Verification items for the finished model (mm, model axes). Face numbers are marked on the shaded views. A direction names the side the tool comes from. Coordinates: 2 decimals unless noted, no trailing zeros. Order: outer loops, then holes, each group sorted by start corner. A loop starts at its lowest first (then second) coordinate and runs counter-clockwise, first axis right, second up. Notation, with made-up numbers: (78, 26) -> (115, 26) arc R6 ccw to (115, 31) -> close; hole circle Ø6 at (56.25, -22.75). An arc over 180 degrees is marked (long way). Write item = value, one per line. Start each with the question number.
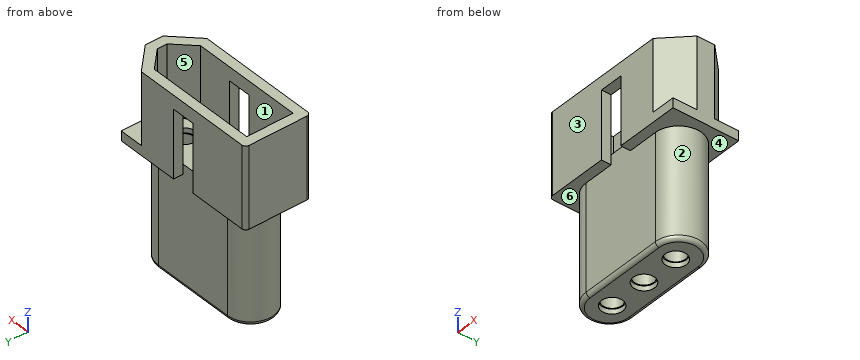
from build123d import *

# Parameters (mm, degrees)
BOSS_EXTRUDE1_DEPTH = 10.668
SKETCH2_R           = 1.27
BOSS_EXTRUDE2_DEPTH = 15.6591
BOSS_EXTRUDE3_START = -1.27
BOSS_EXTRUDE3_DEPTH = 1.27
SKETCH4_R           = 1.397
CUT_EXTRUDE1_DEPTH  = 0.635
CUT_EXTRUDE2_START  = -0.635
SKETCH5_R           = 1.397
CUT_EXTRUDE2_DEPTH  = 0.635
SKETCH6_W           = 3.048
SKETCH6_H           = 1.27
CUT_EXTRUDE3_DEPTH  = 8.89
FILLET1_R           = 0.508


# Read off the part's stored shape, not the designer's step: Boss-Extrude3
with BuildPart() as part:
    # Sketch1 → Boss-Extrude1 (new body)
    with BuildSketch(Plane.XY):
        with BuildLine():
            Line((6.622051224, 4.318), (-9.271, 4.318))
            ThreePointArc((-9.271, 4.318), (-9.630210245, 4.169210245), (-9.779, 3.81))
            Line((-9.779, 3.81), (-9.779, -3.81))
            ThreePointArc((-9.779, -3.81), (-9.630210245, -4.169210245), (-9.271, -4.318))
            Line((-9.271, -4.318), (6.622051224, -4.318))
            Line((6.622051224, -4.318), (9.779, -1.161051224))
            Line((9.779, -1.161051224), (9.779, 1.161051224))
            Line((9.779, 1.161051224), (6.622051224, 4.318))
        make_face()
        Polygon((8.509, -0.635), (8.509, 0.635), (6.096, 3.048), (-8.509, 3.048), (-8.509, -3.048), (6.096, -3.048), align=None, mode=Mode.SUBTRACT)
    extrude(amount=-BOSS_EXTRUDE1_DEPTH)



with BuildPart() as body_2:
    # Sketch2 → Boss-Extrude2 (new body)
    with BuildSketch(Plane.XY.offset(-25.0571)):
        with BuildLine():
            Line((-5.461, 3.048), (5.461, 3.048))
            ThreePointArc((5.461, 3.048), (8.509, 0), (5.461, -3.048))
            Line((5.461, -3.048), (-5.461, -3.048))
            ThreePointArc((-5.461, -3.048), (-8.509, 0), (-5.461, 3.048))
        make_face()
        with Locations((-5.0292, 0)):
            Circle(SKETCH2_R, mode=Mode.SUBTRACT)
        with Locations((5.0292, 0)):
            Circle(SKETCH2_R, mode=Mode.SUBTRACT)
        Circle(SKETCH2_R, mode=Mode.SUBTRACT)
    extrude(amount=BOSS_EXTRUDE2_DEPTH)


with BuildPart() as part_1:
    add(part.part)

    add(body_2.part)  # Boss-Extrude3 merges body 2
    # Boss-Extrude3 outline → Boss-Extrude3 (add)
    with BuildSketch(Plane.XY.offset(-9.398).offset(BOSS_EXTRUDE3_START)):
        Polygon((6.622051224, -4.318), (9.779, -4.318), (9.779, -1.161051224), align=None)
        Polygon((6.622051224, 4.318), (9.779, 1.161051224), (9.779, 4.318), align=None)
        with BuildLine():
            Line((5.461, -3.048), (6.096, -3.048))
            Line((6.096, -3.048), (6.182665302, -2.961334698))
            ThreePointArc((6.182665302, -2.961334698), (5.824425262, -3.026256116), (5.461, -3.048))
        make_face()
        with BuildLine():
            ThreePointArc((8.509, 0), (8.487256116, -0.363425262), (8.422334698, -0.721665302))
            Line((8.422334698, -0.721665302), (8.509, -0.635))
            Line((8.509, -0.635), (8.509, 0))
        make_face()
        with BuildLine():
            Line((-8.509, -3.048), (-5.461, -3.048))
            ThreePointArc((-5.461, -3.048), (-7.616261469, -2.155261469), (-8.509, 0))
            Line((-8.509, 0), (-8.509, -3.048))
        make_face()
        with BuildLine():
            ThreePointArc((8.422334698, 0.721665302), (8.487256116, 0.363425262), (8.509, 0))
            Line((8.509, 0), (8.509, 0.635))
            Line((8.509, 0.635), (8.422334698, 0.721665302))
        make_face()
        with BuildLine():
            Line((-8.509, 3.048), (-8.509, 0))
            ThreePointArc((-8.509, 0), (-7.616261469, 2.155261469), (-5.461, 3.048))
            Line((-5.461, 3.048), (-8.509, 3.048))
        make_face()
        with BuildLine():
            ThreePointArc((5.461, 3.048), (5.824425262, 3.026256116), (6.182665302, 2.961334698))
            Line((6.182665302, 2.961334698), (6.096, 3.048))
            Line((6.096, 3.048), (5.461, 3.048))
        make_face()
    extrude(amount=BOSS_EXTRUDE3_DEPTH)

    # Sketch4 → Cut-Extrude1 (cut)
    with BuildSketch(Plane(origin=(0, 0, -25.0571), x_dir=(-1, 0, 0), z_dir=(0, 0, -1))):
        with Locations((-5.0292, 0)):
            Circle(SKETCH4_R)
        with Locations((5.0292, 0)):
            Circle(SKETCH4_R)
        Circle(SKETCH4_R)
    extrude(amount=-CUT_EXTRUDE1_DEPTH, mode=Mode.SUBTRACT)

    # Sketch5 → Cut-Extrude2 (cut)
    with BuildSketch(Plane.XY.offset(-9.398).offset(CUT_EXTRUDE2_START)):
        with Locations(Location((0, 0, 0), (0, 0, 180))):
            Circle(SKETCH5_R)
        with Locations(Location((-5.0292, 0, 0), (0, 0, 180))):
            Circle(SKETCH5_R)
        with Locations(Location((5.0292, 0, 0), (0, 0, 180))):
            Circle(SKETCH5_R)
    extrude(amount=CUT_EXTRUDE2_DEPTH, mode=Mode.SUBTRACT)

    # Sketch6 → Cut-Extrude3 (cut)
    with BuildSketch(Plane(origin=(0, 0, -10.668), x_dir=(-1, 0, 0), z_dir=(0, 0, -1))):
        with Locations((0, 3.683)):
            Rectangle(SKETCH6_W, SKETCH6_H)
        with Locations((0, -3.683)):
            Rectangle(SKETCH6_W, SKETCH6_H)
    extrude(amount=-CUT_EXTRUDE3_DEPTH, mode=Mode.SUBTRACT)

    # Fillet1
    fillet1_edges = [part_1.edges().sort_by_distance(p)[0] for p in [
        (-8.509, 0, -25.0571),
        (0, 3.048, -25.0571),
        (0, -3.048, -25.0571),
        (8.509, 0, -25.0571),
    ]]
    fillet(fillet1_edges, radius=FILLET1_R)


solid = part_1.part
Item 1: Thickness scan on line 1 (X direction, y = 0, z = -14.25); line 2 (X direction, y = -0.5, z = -8); line 3 (Y direction, x = 0, z = -24.55). Record the ranges inside material, lowest first.
Item 2: Mould release check, pull along Y, two halves, no side actions. Record for the marked faces 1, 2 and 3: pulls with the +Y half, pulls with the -Y half, needs draft (parallel to the pull), parting line crosses it, or undercut.
Item 3: Gauge pin test, flat ends, axial feed: P1, Ø1.4, axis at x = -5, y = -0.5, coming from the +Z side; P2, Ø3.5, axis at x = -5.03, y = 0, coming from the +Z side; P3, Ø2, axis at x = 7.5, z = -19.5, coming from the -Y side; P4, Ø3, axis at y = 2.5, z = -15, coming from the +X side. Record the tip position at first contact, or that the pin passes through.
Item 4: Section check B-B (z = -8.25). Record the boundary of the cut face in (x, y) (3 decimals).
Item 5: Section check D-D (z = -18.25). Record the boundary of the cut face in (x, y), then the cut area to 3 significant figures.
Item 6: Tool access check on the marked faces 4, 5 and 6. Record the directions out of +Z, -Z, +X, -X, +Y, -Y that give a thin tool (end or side, any length) a straight path to the whole face; none if there is none.
Item 7: Section check C-C (x = -5). Record the boundary of the cut face in (y, z), then the cut area to 3 significant figures.
Item 8: Section check A-A (x = 0). Record the boundary of the cut face in (y, z), then the cut area to 3 significant figures.
Filled sheet:
q1.line_1 = -8.51 to -6.3, -3.76 to -1.27, 1.27 to 3.76, 6.3 to 8.51
q1.line_2 = -9.78 to -8.51, 8.51 to 9.78
q1.line_3 = -3.05 to -1.4, 1.4 to 3.05
q2.face_1 = undercut
q2.face_2 = parting line crosses it
q2.face_3 = pulls with the -Y half
q3.P1 = through
q3.P2 = -9.4
q3.P3 = -2.87
q3.P4 = 8.34
q4.outline = (-9.779, -3.81) arc R0.508 ccw to (-9.271, -4.318) -> (-1.524, -4.318) -> (-1.524, -3.048) -> (-8.509, -3.048) -> (-8.509, 3.048) -> (-1.524, 3.048) -> (-1.524, 4.318) -> (-9.271, 4.318) arc R0.508 ccw to (-9.779, 3.81) -> close; (1.524, -4.318) -> (6.622, -4.318) -> (9.779, -1.161) -> (9.779, 1.161) -> (6.622, 4.318) -> (1.524, 4.318) -> (1.524, 3.048) -> (6.096, 3.048) -> (8.509, 0.635) -> (8.509, -0.635) -> (6.096, -3.048) -> (1.524, -3.048) -> close
q5.outline = (-5.46, -3.05) -> (5.46, -3.05) arc R3.05 ccw to (5.46, 3.05) -> (-5.46, 3.05) arc R3.05 ccw to start; hole circle Ø2.54 at (-5.03, 0); hole circle Ø2.54 at (0, 0); hole circle Ø2.54 at (5.03, 0)
q5.area = 80.6 mm^2
q6.face_4 = -Z, +X
q6.face_5 = +Z
q6.face_6 = -Z, -X
q7.outline = (-4.32, -10.67) -> (-3.05, -10.67) -> (-3.05, -24.55) arc R0.51 ccw to (-2.54, -25.06) -> (-1.4, -25.06) -> (-1.4, -24.42) -> (-1.27, -24.42) -> (-1.27, -10.03) -> (-1.4, -10.03) -> (-1.4, -9.4) -> (-3.05, -9.4) -> (-3.05, 0) -> (-4.32, 0) -> close; (1.27, -24.42) -> (1.4, -24.42) -> (1.4, -25.06) -> (2.54, -25.06) arc R0.51 ccw to (3.05, -24.55) -> (3.05, -10.67) -> (4.32, -10.67) -> (4.32, 0) -> (3.05, 0) -> (3.05, -9.4) -> (1.4, -9.4) -> (1.4, -10.03) -> (1.27, -10.03) -> close
q7.area = 82.4 mm^2
q8.outline = (-4.32, -1.78) -> (-3.05, -1.78) -> (-3.05, 0) -> (-4.32, 0) -> close; (-3.05, -24.55) arc R0.51 ccw to (-2.54, -25.06) -> (-1.4, -25.06) -> (-1.4, -24.42) -> (-1.27, -24.42) -> (-1.27, -10.03) -> (-1.4, -10.03) -> (-1.4, -9.4) -> (-3.05, -9.4) -> close; (1.27, -24.42) -> (1.4, -24.42) -> (1.4, -25.06) -> (2.54, -25.06) arc R0.51 ccw to (3.05, -24.55) -> (3.05, -9.4) -> (1.4, -9.4) -> (1.4, -10.03) -> (1.27, -10.03) -> close; (3.05, -1.78) -> (4.32, -1.78) -> (4.32, 0) -> (3.05, 0) -> close
q8.area = 59.8 mm^2
